Work out the finished part from the listing and answer in its coordinate system (mm). Face numbers are marked on the shaded views. A direction names the side the tool comes from. Round coordinates to 2 decimals unless told otherwise and drop trailing zeros. Loops run counter-clockwise (first coordinate to the right, second up) from the corner with the lowest first, then second, coordinate; pieces in that order, holes last. Notation, with made-up numbers: (55.25, -24) - (103.25, -24) arc R29 cw to (103.25, 6) - close; hole circle Ø1 at (85, -2.75). An arc over 180 degrees is marked (long way). Return JSON: item names as keys, results as strings.
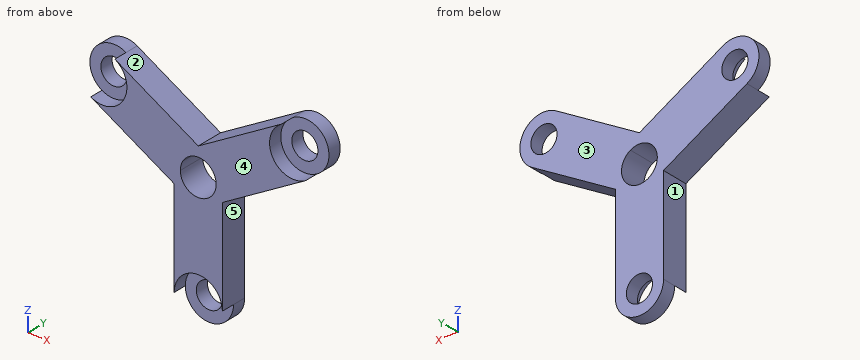
Autodesk Inventor part; units mm, degrees
ref_plane "YZ Plane" through (0, 0, 0) normal (1, 0, 0) x (0, 1, 0)
ref_plane "XZ Plane" through (0, 0, 0) normal (0, 1, 0) x (-1, 0, 0)
ref_plane "XY Plane" through (0, 0, 0) normal (0, 0, 1) x (1, 0, 0)
sketch "Эскиз1" plane through (0, 0, 0) normal (0, 1, 0) x (-1, 0, 0)
  point P0 (0, 0)
sketch "Эскиз2" plane through (0, 0, 0) normal (0, 1, 0) x (-1, 0, 0)
  line L0 (0, 0) -> (0, -16)
  circle A0 centre (0, -16) radius 1.9
  circle A1 centre (0, 0) radius 2.6
  line L1 (0, 0) -> (0, -16) construction
  line L2 (-3.5, 0) -> (-3.5, -16)
  line L3 (3.5, -16) -> (3.5, 0)
  arc A2 (3.5, 0) -> (-3.5, 0) centre (0, 0) ccw
  arc A3 (-3.5, -16) -> (3.5, -16) centre (0, -16) ccw
  point P0 (0, -8)
  dimension "d0" = 16
  dimension "d1" = 3.8
  dimension "d2" = 5.2
  dimension "d3" = 7
extrude "Выдавливание1" add sketch "Эскиз2" along normal blind 4
pattern_circular "Круговой массив1" count 3 over 360 about axis through (0, 0, 0) along (0, 1, 0) of "Выдавливание1"
sketch "Эскиз4" plane through (0, 0, 0) normal (0, -1, 0) x (1, 0, 0)
  circle A0 centre (13.8564, 8) radius 1.9
  line L0 (15.6064, 4.9689) -> (3.5, -2.0207)
  circle A1 centre (13.8564, 8) radius 3.5
  point P0 (0, 0)
extrude "Выдавливание3" cut sketch "Эскиз4" against normal blind 2
pattern_circular "Круговой массив2" count 3 over 360 about axis through (0, 0, 0) along (0, 1, 0) of "Выдавливание3"
properties part number "gearbox_secondary_gear_holder"
1) Section B-B (y = 0.75) is taken. Give the vertices of the cut face in (x, z), and give its area (3 significant figures).
Verdict:
{"outline": "(-15.6, 4.97) - (-3.5, -2.02) - (-3.5, -16) arc R3.5 cw to (3.5, -16) - (3.5, -2.02) - (15.61, 4.97) arc R3.5 cw to (12.1, 11.03) - (0, 4.04) - (-12.11, 11.03) arc R3.5 cw to start; hole circle Ø5.2 at (0, 0)", "area": "236 mm2"}
2) Determine the mould class of the marked faces 3, 4 and 5 for opening direction Y: pulls with the +Y half, pulls with the -Y half, needs draft (parallel to the pull), parting line crosses it, or undercut.
Verdict:
{"face 3": "pulls with the +Y half", "face 4": "pulls with the -Y half", "face 5": "needs draft"}
3) Section C-C (z = -6) is taken. Give the vertices of the cut face in (x, y).
Verdict:
{"outline": "(-3.5, 0) - (3.5, 0) - (3.5, 4) - (-3.5, 4) - close"}
4) Section A-A (z = 8) is taken. Give the vertices of the cut face in (x, y).
Verdict:
{"outline": "(-17.36, 2) - (-15.76, 2) - (-15.76, 4) - (-17.36, 4) - close; (-11.96, 2) - (-10.36, 2) - (-10.36, 0) - (-6.86, 0) - (-6.86, 4) - (-11.96, 4) - close; (6.86, 0) - (10.36, 0) - (10.36, 2) - (11.96, 2) - (11.96, 4) - (6.86, 4) - close; (15.76, 2) - (17.36, 2) - (17.36, 4) - (15.76, 4) - close"}
5) Find the intervals of material crossed by L1, parallel to Z at x = 0, y = 2.9; L2, parallel to X at y = 2.65, z = 8; L3, parallel to X at y = 3.25, z = -6, in increasing order.
Verdict:
{"L1": "z = -19.5 to -17.9, -14.1 to -2.6, 2.6 to 4.04", "L2": "x = -17.36 to -15.76, -11.96 to -6.86, 6.86 to 11.96, 15.76 to 17.36", "L3": "x = -3.5 to 3.5"}
6) Flat-ended cylindrical pins translate along their axes: pin 1 (3 mm diameter, centred on x = -3, z = 6, fed in from +Y); pin 2 (3.5 mm diameter, centred on x = 14, z = 6.5, fed in from -Y); pin 3 (1.2 mm diameter, centred on y = 2.5, z = -8.5, fed in from -X); pin 4 (2 mm diameter, centred on x = -12, y = 2.5, fed in from -Z). Find the tip coordinate at first contact, or state that the pin passes through.
Verdict:
{"pin 1": "stops at y = 4", "pin 2": "stops at y = 2", "pin 3": "stops at x = -3.5", "pin 4": "stops at z = 2.31"}
7) Section D-D (x = -9) is taken. Give the vertices of the cut face in (y, z), and give its area (3 significant figures).
Verdict:
{"outline": "(0, 1.15) - (4, 1.15) - (4, 9.24) - (0, 9.24) - close", "area": "32.3 mm2"}
8) A tool of negligible diameter and unlimited length cuts with its end or side. For the marked faces 1 and 2, from which of +Z, -Z, +X, -X, +Y, -Y can it reach the whole face along a straight path? Write none if from no direction.
Verdict:
{"face 1": "-Z, -X, +Y, -Y", "face 2": "+Z, +Y, -Y"}
